Could you check a few things on this model? Use its own coordinates, in mm. Coordinates: 2 decimals unless noted, no trailing zeros. Order: outer loops, then holes, each group sorted by start corner. A loop starts at its lowest first (then second) coordinate and runs counter-clockwise, first axis right, second up. Notation, with made-up numbers: M 61,-22 L 76,-22 A21 ccw 76,8 Z; hole C -34,3 d5. An arc over 180 degrees is marked long. Write item = value, one per line. Start each with the question number.
from build123d import *

# Parameters (mm, degrees)
SKETCH2_R           = 0.5
BOSS_EXTRUDE1_DEPTH = 15.5
SKETCH2_6_R         = 1.2
SKETCH2_6_R_2       = 0.5
BOSS_EXTRUDE3_DEPTH = 4.75
SKETCH3_R           = 0.5
BOSS_EXTRUDE4_DEPTH = 4.75
FILLET1_R           = 0.2
SKETCH4_R           = 0.85
BOSS_EXTRUDE5_DEPTH = 0.3
SKETCH6_W           = 0.466741821
SKETCH6_H           = 0.031322261
SKETCH7_W           = 1.509947497
SKETCH7_H           = 2.46


with BuildPart() as part:
    # Sketch2 → Boss-Extrude1 (new body)
    with BuildSketch(Plane.XY):
        Circle(SKETCH2_R)
    extrude(amount=BOSS_EXTRUDE1_DEPTH)



with BuildPart() as body_2:
    # Sketch2_6 → Boss-Extrude3 (new body)
    with BuildSketch(Plane.XY):
        Circle(SKETCH2_6_R)
        Circle(SKETCH2_6_R_2, mode=Mode.SUBTRACT)
    extrude(amount=-BOSS_EXTRUDE3_DEPTH)


with BuildPart() as part_1:
    add(part.part)

    add(body_2.part)  # Boss-Extrude4 merges body 2
    # Sketch3 → Boss-Extrude4 (add)
    with BuildSketch(Plane(origin=(0, 0, 0), x_dir=(-1, 0, 0), z_dir=(0, 0, -1))):
        with Locations(Location((0, 0, 0), (0, 0, 180))):
            Circle(SKETCH3_R)
    extrude(amount=BOSS_EXTRUDE4_DEPTH)

    # Fillet1
    fillet1_edges = [part_1.edges().sort_by_distance(p)[0] for p in [
        (-1.2, 0, 0),
    ]]
    fillet(fillet1_edges, radius=FILLET1_R)

    # Sketch4 → Boss-Extrude5 (add)
    with BuildSketch(Plane.XY):
        Circle(SKETCH4_R)
    extrude(amount=BOSS_EXTRUDE5_DEPTH)

    # Sketch5 → Revolve1 (revolve)
    with BuildSketch(Plane(origin=(0, 0, 0), x_dir=(1, 0, 0), z_dir=(0, 1, 0)), mode=Mode.PRIVATE) as revolve1_sk:
        with BuildLine():
            Line((0.5, -15.5), (0, -15.5))
            Line((0, -15.5), (0, -16.0775))
            ThreePointArc((0, -16.0775), (0.247487373, -16.180012627), (0.35, -16.4275))
            Line((0.35, -16.4275), (0.5, -16.4275))
            ThreePointArc((0.5, -16.4275), (0.44489867, -16.199322057), (0.291739306, -16.021435747))
            Line((0.291739306, -16.021435747), (0.291739306, -15.774240314))
            Line((0.291739306, -15.774240314), (0.524883028, -15.774240314))
            Line((0.524883028, -15.774240314), (0.524883028, -15.652417135))
            Line((0.524883028, -15.652417135), (0.376771599, -15.652417135))
            ThreePointArc((0.376771599, -15.652417135), (0.411432347, -15.554416852), (0.5, -15.5))
        make_face()
    revolve(revolve1_sk.sketch.rotate(Axis((0, 0, 15.5), (0, 0, 1)), 180), axis=Axis((0, 0, 15.5), (0, 0, 1)))

    # Sketch6 → Revolve2 (revolve)
    with BuildSketch(Plane(origin=(0, 0, 0), x_dir=(1, 0, 0), z_dir=(0, 1, 0))):
        with Locations((-0.233370911, -16.32433887)):
            Rectangle(SKETCH6_W, SKETCH6_H)
    revolve(axis=Axis((0, 0, 16.4275), (0, 0, -1)))

    # Sketch7 → Cut-Revolve1 (revolve, cut)
    with BuildSketch(Plane(origin=(0, 0, 0), x_dir=(1, 0, 0), z_dir=(0, 1, 0))):
        with Locations((-1.051173749, -14.27)):
            Rectangle(SKETCH7_W, SKETCH7_H)
    revolve(axis=Axis((0, 0, 15.5), (0, 0, 1)), mode=Mode.SUBTRACT)


solid = part_1.part
(1) Please list where these lines run through material, in increasing order: probe 1 along Z at (x, y) = (0.25, -0.95); probe 2 along Z at (x, y) = (-0.2, -0.65); probe 3 along X at (y, z) = (-0.4, 4.75). Write a range as from..to.
(2) Imagine slicing it at A-A on z = -2.75. List the corners of the cut face in (x, y) for me.
(3) Will this pin go through, and if not, where does the flat tip stop? P1, Ø1, axis at y = 0, z = 7.5, coming from the +X side.
(4) Thinking about a two-plate mould opening in Z: for faces 1 (the cylindrical face through (-0.108, -0.488, 6.581)), 2 (the cylindrical face through (0.65, 1.01, -2.44)), 3 (the flat face through (0, 0, -4.75)), which applies, released by +Z, released by -Z, zero draft, split by the parting line, or undercut?
(5) Imagine slicing it at B-B on z = 11.25. List the corners of the cut face in (x, y) for me.
Response:
q1.probe_1 = -4.75..0
q1.probe_2 = -4.75..0.3
q1.probe_3 = -0.3..0.3
q2.outline = C 0,0 d2.4
q3.P1 = 0.5
q4.face_1 = undercut
q4.face_2 = zero draft
q4.face_3 = released by -Z
q5.outline = C 0,0 d1
